```python
from build123d import *

# Parameters (mm, degrees)
F0_R     = 15
F0_R_2   = 11.025
F3_DEPTH = 25
F2_R     = 11.025
F4_DEPTH = 40.1
F6_DEPTH = 15
F7_DEPTH = 7
F8_DEPTH = 2.9


# Not quite as in the source:
# - ends of sketch curves that miss each other by under 0.0002 mm in the source are joined


with BuildPart() as f3:
    # F0 (on Front) → F3 (new body)
    with BuildSketch(Plane.XZ):
        Circle(F0_R)
        Circle(F0_R_2, mode=Mode.SUBTRACT)
    extrude(amount=F3_DEPTH)


with BuildPart() as f3b:
    # F1 (on Front) → F3, piece 2 (new body)
    with BuildSketch(Plane.XZ):
        Polygon((0, 24.356296724), (-6.821225702, 13.2896405025), (-6.821225702, 0), (0, 0), (6.821225702, 0), (6.821225702, 13.2896405025), align=None)
        Polygon((0, 0), (-6.821225702, 0), (-6.821225702, -10.4577671736), (-6.82123, -10.4854255915), (-6.821225702, -13.2896405025), (0, -24.356296724), (6.821225702, -13.2896405025), (6.821225702, 0), align=None)
    extrude(amount=F3_DEPTH)

    # F2 (on face) → F4 (cut)
    with BuildSketch(Plane.XZ):
        Circle(F2_R)
    extrude(amount=F4_DEPTH, mode=Mode.SUBTRACT)

    # F5: union F3
    add(f3.part)

    # F6 (cut): a face of the model
    f6_faces = [f3b.faces().sort_by_distance(p)[0] for p in [
        (-11.5970941147, -25, 0),
    ]]
    extrude(f6_faces, amount=-F6_DEPTH, mode=Mode.SUBTRACT)

    # F7 (cut): a face of the model
    f7_faces = [f3b.faces().sort_by_distance(p)[0] for p in [
        (-11.5970941147, 0, 0),
    ]]
    extrude(f7_faces, amount=-F7_DEPTH, mode=Mode.SUBTRACT)

    # F8 (add): a face of the model
    f8_faces = [f3b.faces().sort_by_distance(p)[0] for p in [
        (-11.5970941147, -10, 0),
    ]]
    extrude(f8_faces, amount=F8_DEPTH)


solid = f3b.part
```
Source: CAD feature listing. Evaluate the final solid. Frame: model axes, mm. Coordinates: 2 decimals unless noted, no trailing zeros. Loops run counter-clockwise (first coordinate to the right, second up) from the corner with the lowest first, then second, coordinate; pieces in that order, holes last. Notation, with made-up numbers: (23, -15) -> (73, -15) arc R10 cw to (73, -5) -> close; hole circle Ø4 at (-2, -18.75). An arc over 180 degrees is marked (long way). One line per item, written item: value. Start each with the question number.
Q1. Section query C-C, the plane x = -5.25. Return the cut outline in (y, z), and give its area (3 significant figures).
Q2. Line query: line 1 along Z through (x, y) = (-2.5, -10.4); line 2 along Z through (x, y) = (-9.75, -8.45); line 3 along X through (y, z) = (-10.45, -3.5). Output: solid intervals per line, ascending.
Q3. Section query B-B, the plane y = -11.75. Return the cut outline in (x, z) (3 decimals).
Q4. Contact query for flat-ended pins moving along their axis: P1, Ø1.5, axis at x = 8.5, y = -10, coming from the -Z side; P2, Ø1.5, axis at x = 2.5, y = -10, coming from the -Z side; P3, Ø2, axis at x = -8.5, y = -10, coming from the +Z side; P4, Ø4, axis at x = 7.5, z = 2, coming from the -Y side. Output: stop coordinate, or through.
Q5. Mould query, pull axis Z, two halves, no side actions, for faces 1 (the face through (-11, -12.9, -2)), 2 (the face through (15, -10, 0)), 3 (the face through (-2.39, -9.909, 10.763)). Classes: pulls with the +Z half, pulls with the -Z half, needs draft (parallel to the pull), parting line crosses it, or undercut.
Q6. Section query A-A, the plane z = 0. Return the cut outline in (x, y) (3 decimals), and give its area (3 significant figures).
Q7. Section query D-D, the plane z = -12. Return the cut outline in (x, y), and give its area (3 significant figures).
Results:
1. outline: (-12.9, -15.84) -> (-7, -15.84) -> (-7, -9.69) -> (-12.9, -9.69) -> close; (-12.9, 9.69) -> (-7, 9.69) -> (-7, 15.84) -> (-12.9, 15.84) -> close
1. area: 72.5 mm^2
2. line 1: -20.3 to -10.74, 10.74 to 20.3
2. line 2: -11.4 to -5.15, 5.15 to 11.4
2. line 3: -14.59 to -10.45, 10.45 to 14.59
3. outline: (-6.759, -13.391) -> (0, -24.356) -> (6.759, -13.391) arc R15 ccw to (6.759, 13.391) -> (0, 24.356) -> (-6.759, 13.391) arc R15 ccw to start; hole circle Ø22.05 at (0, 0)
4. P1: z = -12.84
4. P2: z = -21.52
4. P3: z = 12.99
4. P4: through
5. face 1: needs draft
5. face 2: parting line crosses it
5. face 3: undercut
6. outline: (-15, -12.9) -> (-11.025, -12.9) -> (-11.025, -7) -> (-15, -7) -> close; (11.025, -12.9) -> (15, -12.9) -> (15, -7) -> (11.025, -7) -> close
6. area: 46.9 mm^2
7. outline: (-9, -12.9) -> (9, -12.9) -> (9, -7) -> (-9, -7) -> close
7. area: 106 mm^2
